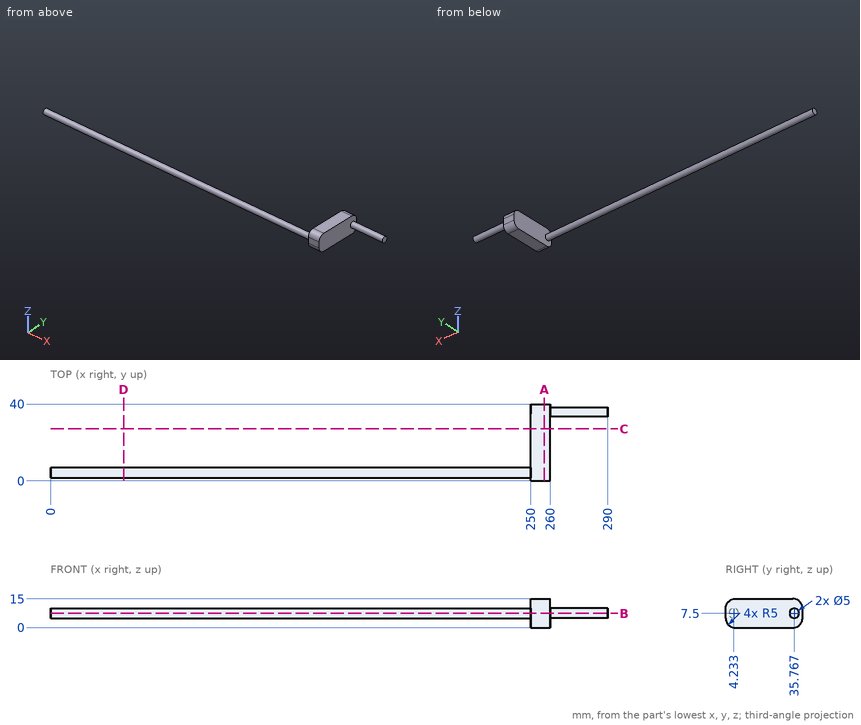
Here's the drawing with two shaded views (mm, measured from the low corner). I have some questions. Round coordinates to 2 decimals unless told otherwise and drop trailing zeros. Loops run counter-clockwise (first coordinate to the right, second up) from the corner with the lowest first, then second, coordinate; pieces in that order, holes last.
Item 1: Please list where these lines run through material, in increasing order: L1, parallel to X at y = 9.5, z = 3.75; L2, parallel to Y at x = 28.5, z = 7.25; L3, parallel to Z at x = 79, y = 4.
Item 2: Suppose I cut it at C-C, the plane y = 27. Write out the boundary of the cut face in (x, z).
Item 3: Suppose I cut it at D-D, the plane x = 38. Write out the boundary of the cut face in (y, z).
Item 4: Suppose I cut it at B-B, the plane z = 7.5. Write out the boundary of the cut face in (x, y).
Item 5: Will these pins go through, and if not, where does the flat tip stop? pin 1 Ø7.5 at (y, z) = (18, 8) entering from +X; pin 2 Ø8 at (y, z) = (31, 12) entering from -X; pin 3 Ø1 at (x, z) = (184, 8.5) entering from -Y.
Item 6: Suppose I cut it at A-A, the plane x = 257. Write out the boundary of the cut face in (y, z).
Reported:
1. L1: x = 250 to 260
1. L2: y = 1.75 to 6.72
1. L3: z = 5.01 to 9.99
2. outline: (250, 0) - (260, 0) - (260, 15) - (250, 15) - close
3. outline: circle Ø5 at (4.23, 7.5)
4. outline: (0, 1.73) - (250, 1.73) - (250, 0) - (260, 0) - (260, 33.27) - (290, 33.27) - (290, 38.27) - (260, 38.27) - (260, 40) - (250, 40) - (250, 6.73) - (0, 6.73) - close
5. pin 1: stops at x = 260
5. pin 2: stops at x = 250
5. pin 3: stops at y = 1.78
6. outline: (0, 5) arc R5 ccw to (5, 0) - (35, 0) arc R5 ccw to (40, 5) - (40, 10) arc R5 ccw to (35, 15) - (5, 15) arc R5 ccw to (0, 10) - close
